Part model, mm, in its own coordinate system. Face numbers are marked on the shaded views. Round coordinates to 2 decimals unless told otherwise and drop trailing zeros. Loops run counter-clockwise (first coordinate to the right, second up) from the corner with the lowest first, then second, coordinate; pieces in that order, holes last. Notation, with made-up numbers: M -38,10.5 L -30,10.5 A12 ccw -30,26.5 Z; hole C -33.5,68.5 d5. An arc over 180 degrees is marked long. Put each result on its own line as item: value. Start each with the question number.
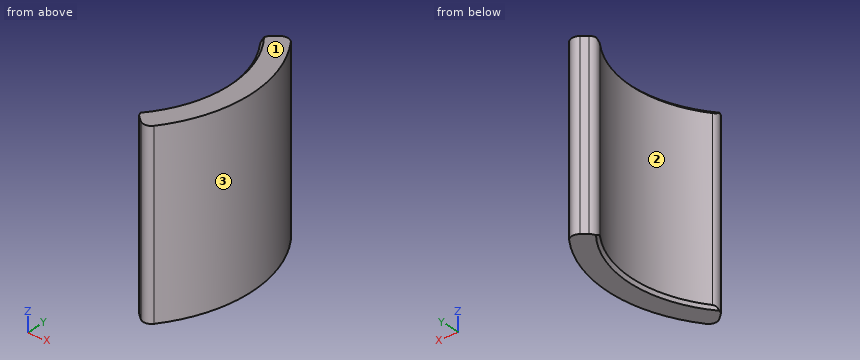
```python
from build123d import *

# Parameters (mm, degrees)
EXTRUSION1_DEPTH = 64
CHANFREIN1_SIZE  = 1
CONG_1_R         = 3


with BuildPart() as part:
    # Esquisse1 → Extrusion1 (new body)
    with BuildSketch(Plane.XY):
        with BuildLine():
            Line((49, 0), (40.5, 0))
            ThreePointArc((40.5, 0), (38.05755114182933, 13.851815804689483), (31.024799946318748, 26.032898192304682))
            Line((31.024799946318748, 26.032898192304682), (37.53617771283009, 31.496592874640232))
            ThreePointArc((37.53617771283009, 31.496592874640232), (46.04493841850956, 16.758987022957648), (49, 0))
        make_face()
    extrusion1 = extrude(amount=EXTRUSION1_DEPTH)

    # Symétrie1: Extrusion1 across plane
    add(extrusion1.mirror(Plane(origin=(49, 0, 64), x_dir=(0, 0, 1), z_dir=(0, 1, 0))))

    # Chanfrein1
    chanfrein1_edges = [part.edges().sort_by_distance(p)[0] for p in [
        (40.50000000000001, 3.55e-15, 64),
        (40.50000000000001, -3.55e-15, 0),
    ]]
    chamfer(chanfrein1_edges, length=CHANFREIN1_SIZE)

    # Congé1
    cong_1_edges = [part.edges().sort_by_distance(p)[0] for p in [
        (31.02479994631875, 26.032898192304682, 32),
        (37.536177712830096, 31.496592874640232, 32),
        (37.536177712830096, -31.496592874640232, 32),
        (31.02479994631875, -26.032898192304682, 32),
    ]]
    fillet(cong_1_edges, radius=CONG_1_R)


solid = part.part
```
1. Drop flat-ended pins along their axis: pin 1 (1 mm diameter, centred on y = -5.5, z = 7, fed in from -X); pin 2 (1.5 mm diameter, centred on y = 22.5, z = 38.5, fed in from +X); pin 3 (4 mm diameter, centred on x = 40.5, z = 7.5, fed in from +Y). Give the stop position or say it passes through.
2. Cut at B-B, the plane x = 47.5. Give the cut face in (y, z), and give its area (3 significant figures).
3. Cut at C-C, the plane x = 43.75. Give the cut face in (y, z).
4. Wall check: L1, parallel to Y at x = 34.25, z = 31.5; L2, parallel to X at y = -1, z = 30; L3, parallel to X at y = -4, z = 38. Give the ranges that are in metal, low to high.
5. Cut at A-A, the plane z = 45. Give the cut face in (x, y), and give its area (3 significant figures).
6. Mould opens along Y. For the marked faces 1, 2 and 3 say: released by +Y, released by -Y, zero draft, split by the parting line, or undercut.
Results list:
1. pin 1: stops at x = 40.05
1. pin 2: stops at x = 43.91
1. pin 3: stops at y = 29.86
2. outline: M -12.03,0 L 12.03,0 L 12.03,64 L -12.03,64 Z
2. area: 1,540 mm^2
3. outline: M -22.07,0 L 22.07,0 L 22.07,64 L -22.07,64 Z
4. L1: y = -28.74 to -21.61, 21.61 to 28.74
4. L2: x = 40.49 to 48.99
4. L3: x = 40.3 to 48.84
5. outline: M 32.75,-23.83 A3 ccw 33.24,-27.89 L 35.16,-29.51 A3 ccw 39.51,-28.98 A49 ccw 39.51,28.98 A3 ccw 35.16,29.51 L 33.24,27.89 A3 ccw 32.75,23.83 A40.5 cw Z
5. area: 523 mm^2
6. face 1: zero draft
6. face 2: undercut
6. face 3: split by the parting line
